Could you check a few things on this drawing? It's one solid part, dimensions in mm from its lowest x, y, z. Round coordinates to 2 decimals unless told otherwise and drop trailing zeros. Loops run counter-clockwise (first coordinate to the right, second up) from the corner with the lowest first, then second, coordinate; pieces in that order, holes last. Notation, with made-up numbers: (54.5, 84.5) -> (75.5, 84.5) arc R16 cw to (75.5, 94.5) -> close; hole circle Ø6 at (-10.75, 55.25). An arc over 180 degrees is marked (long way). Write each question's results on one line, items separated by ' | '.
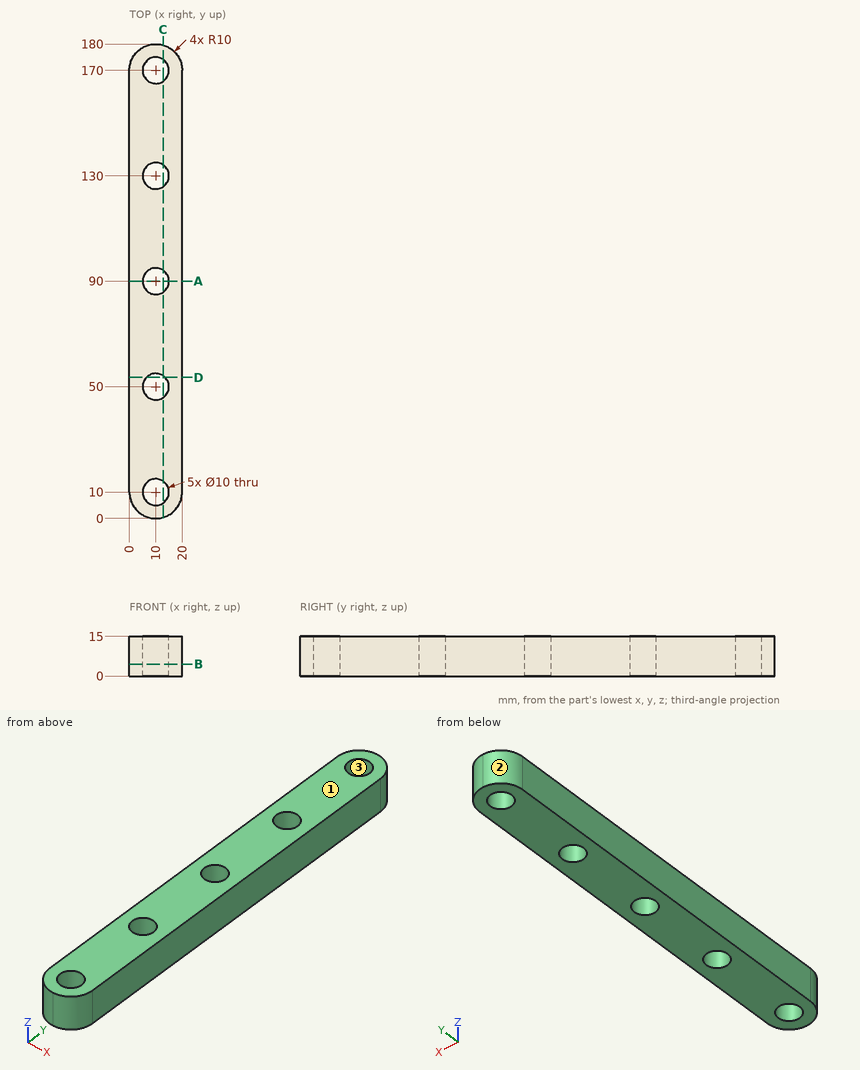
1) I'm going to push flat-ended pins straight in: pin 1 (12 mm diameter, centred on x = 16.5, y = 81.5, fed in from -Z); pin 2 (5 mm diameter, centred on x = 5, z = 5, fed in from +Y). Where does each tip first touch, or does it pass through?
Model answer:
pin 1: stops at z = 0 | pin 2: stops at y = 179.68
2) I want a section at C-C, the plane x = 12.75. Write out the boundary of the cut face in (y, z).
Model answer:
outline: (0.39, 0) -> (5.82, 0) -> (5.82, 15) -> (0.39, 15) -> close; (14.18, 0) -> (45.82, 0) -> (45.82, 15) -> (14.18, 15) -> close; (54.18, 0) -> (85.82, 0) -> (85.82, 15) -> (54.18, 15) -> close; (94.18, 0) -> (125.82, 0) -> (125.82, 15) -> (94.18, 15) -> close; (134.18, 0) -> (165.82, 0) -> (165.82, 15) -> (134.18, 15) -> close; (174.18, 0) -> (179.61, 0) -> (179.61, 15) -> (174.18, 15) -> close
3) I want a section at D-D, the plane y = 53.5. Write out the boundary of the cut face in (x, z).
Model answer:
outline: (0, 0) -> (6.43, 0) -> (6.43, 15) -> (0, 15) -> close; (13.57, 0) -> (20, 0) -> (20, 15) -> (13.57, 15) -> close
4) I need wall thicknesses on line 1 (Y direction, x = 10, z = 7.5); line 2 (X direction, y = 50.5, z = 7) (3 decimals); line 3 (Y direction, x = 11, z = 5.25). Which ranges of each line are inside material? Lowest first, please.
Model answer:
line 1: y = 0 to 5, 15 to 45, 55 to 85, 95 to 125, 135 to 165, 175 to 180 | line 2: x = 0 to 5.025, 14.975 to 20 | line 3: y = 0.05 to 5.1, 14.9 to 45.1, 54.9 to 85.1, 94.9 to 125.1, 134.9 to 165.1, 174.9 to 179.95
5) I want a section at B-B, the plane z = 4.5. Give the number of separate pieces and of enclosed holes in the cut face, plus the area to 3 significant figures.
Model answer:
separate pieces: 1 | enclosed holes: 5 | area: 3,120 mm2
6) If we mould it in two halves opening along Y, with no side actions, what happens to the marked faces 1, 2 and 3? For each: released by +Y, released by -Y, zero draft, split by the parting line, or undercut.
Model answer:
face 1: zero draft | face 2: released by +Y | face 3: undercut
7) I want a section at A-A, the plane y = 90. Write out the boundary of the cut face in (x, z).
Model answer:
outline: (0, 0) -> (5, 0) -> (5, 15) -> (0, 15) -> close; (15, 0) -> (20, 0) -> (20, 15) -> (15, 15) -> close
